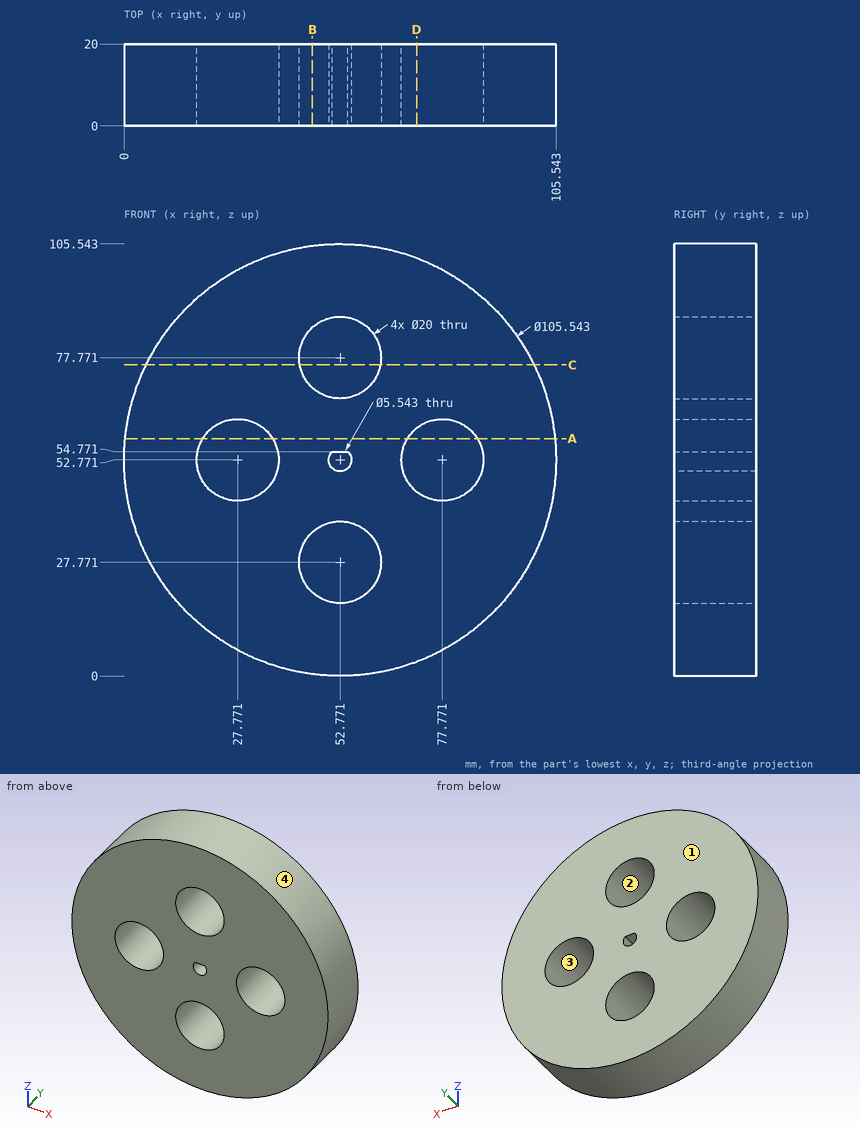
Study the drawing (mm; zero at the part's minimum x, y, z) and answer. Round coordinates to 2 decimals unless told otherwise and drop trailing zeros. Write each loop counter-clockwise with the first axis right and the second up, starting at its lowest first coordinate (ties: lowest second). Pieces come first, ordered by that corner, then holes. Notation, with made-up numbers: (5, 8) - (40, 8) arc R10 cw to (40, 27) - close; hole circle Ø2 at (-28.5, -23.5). An arc over 180 degrees is marked (long way). Use a Markdown table: item, result. Add a question column.
1. The part is cut by section B-B (x = 46). Write down the section's boundary in (y, z).
2. Flat-ended cylindrical pins translate along their axes: P1, Ø1, axis at x = 26.5, z = 77.5, coming from the -Y side; P2, Ø10, axis at x = 14.5, y = 5, coming from the +Z side; P3, Ø1, axis at x = 60.5, y = 10, coming from the -Z side; P4, Ø10, axis at x = 63.5, y = 15, coming from the -Z side. Find the tip coordinate at first contact, or state that the pin passes through.
3. The part is cut by section D-D (x = 71.5). Write down the section's boundary in (y, z) (1 decimal).
4. The part is cut by section A-A (z = 58). Write down the section's boundary in (x, y) (1 decimal).
5. The part is cut by section C-C (z = 76). Write down the section's boundary in (x, y) (1 decimal), and give its area (3 significant figures).
6. Consider line 1 (X direction, y = 18.25, z = 55) (1 decimal); line 2 (X direction, y = 7, z = 55.5); line 3 (Z direction, x = 57, y = 12). Determine where each line is inside the solid, lowest interval first.
7. For a pull along Z with two mould halves and no side action, classify the marked faces 1, 2, 3 and 4 as +Z half, -Z half, draft (parallel to the pull), parting line (faces both ways), or undercut.
Reported:
| question | item | result |
|---|---|---|
| 1 | outline | (0, 0.44) - (20, 0.44) - (20, 20.41) - (0, 20.41) - close; (0, 35.13) - (20, 35.13) - (20, 70.41) - (0, 70.41) - close; (0, 85.13) - (20, 85.13) - (20, 105.11) - (0, 105.11) - close |
| 2 | P1 | y = 0 |
| 2 | P2 | z = 93.73 |
| 2 | P3 | z = 0.5 |
| 2 | P4 | z = 0.31 |
| 3 | outline | (0, 3.4) - (20, 3.4) - (20, 45) - (0, 45) - close; (0, 60.6) - (20, 60.6) - (20, 102.1) - (0, 102.1) - close |
| 4 | outline | (0.3, 0) - (19.2, 0) - (19.2, 20) - (0.3, 20) - close; (36.3, 0) - (69.2, 0) - (69.2, 20) - (36.3, 20) - close; (86.3, 0) - (105.3, 0) - (105.3, 20) - (86.3, 20) - close |
| 5 | outline | (5.4, 0) - (42.9, 0) - (42.9, 20) - (5.4, 20) - close; (62.6, 0) - (100.2, 0) - (100.2, 20) - (62.6, 20) - close |
| 5 | area | 1,500 mm^2 |
| 6 | line 1 | 0 to 18, 37.5 to 68, 87.5 to 105.5 |
| 6 | line 2 | 0.07 to 18.15, 37.39 to 68.15, 87.39 to 105.47 |
| 6 | line 3 | 0.17 to 18.71, 36.83 to 68.71, 86.83 to 105.37 |
| 7 | face 1 | draft |
| 7 | face 2 | undercut |
| 7 | face 3 | undercut |
| 7 | face 4 | parting line |
